The figure shows three views and two pictorial views of one solid part (mm, origin at its lowest corner). Answer the questions. A direction names the side the tool comes from. Round coordinates to 2 decimals unless told otherwise and drop trailing zeros. Write each loop counter-clockwise with the first axis right and the second up, starting at its lowest first coordinate (ties: lowest second). Pieces come first, ordered by that corner, then holes.
Item 1: Find the intervals of material crossed by probe 1 along Z at (x, y) = (5.5, 7.75); probe 2 along X at (y, z) = (11, 17.5); probe 3 along Y at (x, z) = (11.25, 8.75) (1 decimal), in increasing order.
Item 2: Each of these flat-tipped pins is pushed along its axis until it touches: pin 1 (2 mm diameter, centred on y = 3, z = 11, fed in from +X); pin 2 (3 mm diameter, centred on x = 12.5, y = 7.5, fed in from -Z); pin 3 (3 mm diameter, centred on y = 4, z = 7, fed in from +X). Where does it stop, or does it pass through?
Item 3: For a pull along X with two mould halves and no side action, classify the marked faces 1, 2 and 3 as +X half, -X half, draft (parallel to the pull), parting line (faces both ways), or undercut.
Item 4: Find section B-B on x = 20. Give the vertices of the cut face in (y, z) (1 decimal).
Item 5: Find section C-C on z = 14. Give the vertices of the cut face in (x, y).
Item 6: Find section A-A on z = 1.5. Give the vertices of the cut face in (x, y), then the cut area to 3 significant figures.
Item 7: A tool of negligible diameter and unlimited length cuts with its end or side. For the marked faces 4, 5 and 6, from which of +Z, -Z, +X, -X, +Y, -Y can it reach the whole face along a straight path? Write none if from no direction.
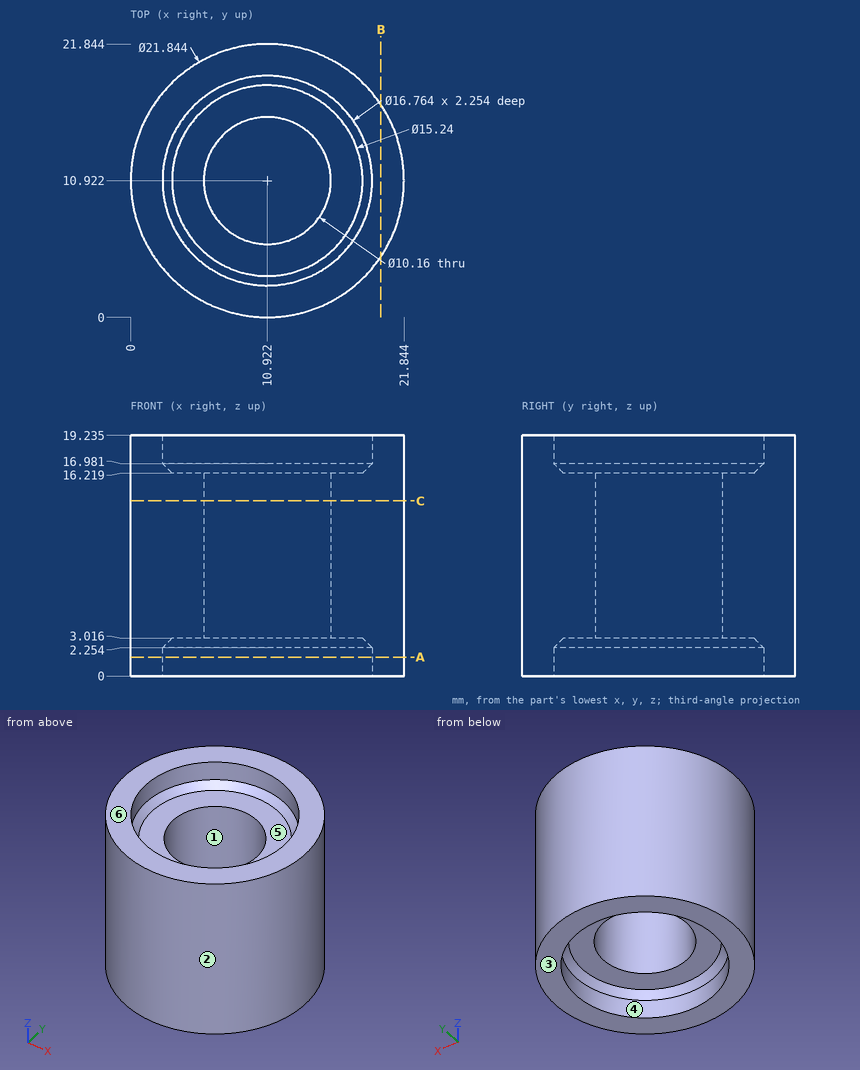
Check values:
1. probe 1: z = 3.02 to 16.22
1. probe 2: x = 0 to 2.54, 19.3 to 21.84
1. probe 3: y = 0 to 5.9, 16 to 21.8
2. pin 1: stops at x = 19.37
2. pin 2: stops at z = 3.02
2. pin 3: stops at x = 20.4
3. face 1: undercut
3. face 2: parting line
3. face 3: draft
4. outline: (4.8, 0) - (17, 0) - (17, 19.2) - (4.8, 19.2) - close
5. outline: circle Ø21.84 at (10.92, 10.92); hole circle Ø10.16 at (10.92, 10.92)
6. outline: circle Ø21.84 at (10.92, 10.92); hole circle Ø16.76 at (10.92, 10.92)
6. area: 154 mm2
7. face 4: -Z
7. face 5: +Z
7. face 6: +Z, +X, -X, +Y, -Y
